Build history of the part. All positions in model axes, mm. Give positions to 0.01 mm unless a question says otherwise; leave off trailing zeros. Write each loop counter-clockwise with the first axis right and the second up, starting at its lowest first coordinate (ties: lowest second). Pieces come first, ordered by that corner, then holes.
from build123d import *

# Parameters (mm, degrees)
F0_R     = 5
F1_DEPTH = 8


with BuildPart() as f1:
    # F0 (on Top) → F1 (new body)
    with BuildSketch(Plane.XY):
        Polygon((8, -4.618802), (8, 4.618802), (0, 9.237604), (-8, 4.618802), (-8, -4.618802), (0, -9.237604), align=None)
        Circle(F0_R, mode=Mode.SUBTRACT)
    extrude(amount=F1_DEPTH)

    # F2 (on Right) → F3 (revolve, intersect)
    with BuildSketch(Plane.YZ):
        Polygon((-8, 0), (0, 0), (0, 8), (-8, 8), (-9.237604, 7.549549), (-9.237604, 0.450451), align=None)
    revolve(axis=Axis((0, 0, 4.732898), (0, 0, 1)), mode=Mode.INTERSECT)


solid = f1.part
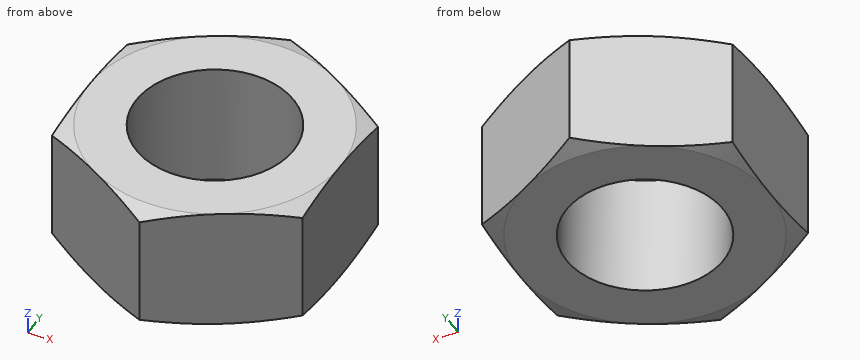
(1) Drop flat-ended pins along their axis: pin 1 (8 mm diameter, centred on x = 0, y = 0, fed in from -Z); pin 2 (2 mm diameter, centred on y = 7, z = 2.5, fed in from -X). Give the stop position or say it passes through.
(2) Saw through at A-A, the plane z = 6.5. List the corners of the cut face in (x, y), plus the area to 3 significant figures.
(3) Probe line 1 (Y direction, x = 3.5, z = 1.75); line 2 (Y direction, x = 0.25, z = 4); line 3 (X direction, y = -2.5, z = 1.25). List the from-to ranges inside material, lowest first.
Computed values:
1. pin 1: passes through
1. pin 2: stops at x = -5.61
2. outline: (-8, -4.62) - (0, -9.24) - (8, -4.62) - (8, 4.62) - (0, 9.24) - (-8, 4.62) - close; hole circle Ø10 at (0, 0)
2. area: 143 mm2
3. line 1: y = -7.22 to -3.57, 3.57 to 7.22
3. line 2: y = -9.09 to -4.99, 4.99 to 9.09
3. line 3: x = -8 to -4.33, 4.33 to 8
